from build123d import *

# Parameters (mm, degrees)
F0_W     = 107.8754812479
F0_H     = 26.1090872809
F1_DEPTH = 12.7
F2_DEPTH = 12.7
F3_R     = 11.2223896829
F4_DEPTH = 177.8
F5_DEPTH = 25.4


with BuildPart() as f1:
    # F0 (on Front) → F1 (new body)
    with BuildSketch(Plane.XZ):
        with Locations((0.7920116186, 0.3961385228)):
            Rectangle(F0_W, F0_H)
    extrude(amount=F1_DEPTH)

    # F2 (add): a face of the model
    f2_faces = [f1.faces().sort_by_distance(p)[0] for p in [
        (0.7920116186, 0, 0.3961385228),
    ]]
    extrude(f2_faces, amount=F2_DEPTH)

    # F3 (on face) → F4 (join)
    with BuildSketch(Plane(origin=(0, 0, -12.6584051177), x_dir=(1, 0, 0), z_dir=(0, 0, -1))):
        Circle(F3_R)
    extrude(amount=F4_DEPTH)

    # F5 (cut): a face of the model
    f5_faces = [f1.faces().sort_by_distance(p)[0] for p in [
        (0.7920116186, -12.7, 0.3961385228),
    ]]
    extrude(f5_faces, amount=-F5_DEPTH, mode=Mode.SUBTRACT)


solid = f1.part
Geometry: final body of the model. Coordinates: model frame, mm. Give positions to 0.01 mm unless a question says otherwise; leave off trailing zeros. Write each loop counter-clockwise with the first axis right and the second up, starting at its lowest first coordinate (ties: lowest second). Pieces come first, ordered by that corner, then holes. Notation, with made-up numbers: (-12.5, 24.25) -> (27.5, 24.25) arc R25 ccw to (27.5, 60.25) -> close; hole circle Ø5 at (-5.75, -5.75). An arc over 180 degrees is marked (long way). Answer as a JSON object with one key per item and string values.
1. Ray query, probe 1 along Y at (x, z) = (-0.75, -51); probe 2 along X at (y, z) = (10, -32.5); probe 3 along X at (y, z) = (-9.25, -154). Return the intervals inside material, ascending. Write a range as from..to.
Ans:
{"probe 1": "y = -11.2..11.2", "probe 2": "x = -5.09..5.09", "probe 3": "x = -6.35..6.35"}
2. Cut plane B-B on x = -7.25. Output: boundary loops of the cut face in (y, z), and give its area (3 significant figures).
Ans:
{"outline": "(-8.57, -190.46) -> (8.57, -190.46) -> (8.57, -12.66) -> (-8.57, -12.66) -> close", "area": "3,050 mm^2"}
3. Contact query for flat-ended pins moving along their axis: pin 1 (1 mm diameter, centred on y = -7, z = -153.5, fed in from -X); pin 2 (2 mm diameter, centred on x = 8, z = -52.5, fed in from +Y); pin 3 (6 mm diameter, centred on x = -6.5, z = -144, fed in from -Y). Output: stop coordinate, or through.
Ans:
{"pin 1": "stops at x = -9.15", "pin 2": "stops at y = 8.77", "pin 3": "stops at y = -10.66"}
4. Cut plane C-C on y = -2. Output: boundary loops of the cut face in (x, z).
Ans:
{"outline": "(-11.04, -190.46) -> (11.04, -190.46) -> (11.04, -12.66) -> (-11.04, -12.66) -> close"}
5. Cut plane A-A on z = -146.5. Output: boundary loops of the cut face in (x, y).
Ans:
{"outline": "circle Ø22.44 at (0, 0)"}
